from build123d import *

# Parameters (mm, degrees)
SKETCH1_R           = 25
BOSS_EXTRUDE1_DEPTH = 15
CUT_EXTRUDE1_DEPTH  = 150
SKETCH3_R           = 1.5
CUT_EXTRUDE2_DEPTH  = 44.660622991
CUT_EXTRUDE3_START  = -7.5
SKETCH4_R           = 2.5
CUT_EXTRUDE3_DEPTH  = 10
CIRPATTERN1_COUNT   = 3
SKETCH5_R           = 2.5
CUT_EXTRUDE4_DEPTH  = 39.405728909


with BuildPart() as part:
    # Sketch1 → Boss-Extrude1 (new body)
    with BuildSketch(Plane(origin=(0, 0, 0), x_dir=(1, 0, 0), z_dir=(0, 1, 0))):
        with Locations(Location((0, 0, 0), (0, 0, 270))):
            Circle(SKETCH1_R)
    extrude(amount=BOSS_EXTRUDE1_DEPTH)

    # Sketch2 → Cut-Extrude1 (cut)
    with BuildSketch(Plane(origin=(0, 15, 0), x_dir=(1, 0, 0), z_dir=(0, 1, 0))):
        with BuildLine():
            Line((7.5, -10), (-7.5, -10))
            Line((-7.5, -10), (-7.5, -23.848480035))
            ThreePointArc((-7.5, -23.848480035), (0, -25), (7.5, -23.848480035))
            Line((7.5, -23.848480035), (7.5, -10))
        make_face()
    cut_extrude1 = extrude(amount=-CUT_EXTRUDE1_DEPTH, mode=Mode.SUBTRACT)

    # Sketch3 → Cut-Extrude2 (cut, symmetric)
    with BuildSketch(Plane.ZY.offset(-7.5)):
        with Locations((16.924240018, 7.5)):
            Circle(SKETCH3_R)
    cut_extrude2 = extrude(amount=CUT_EXTRUDE2_DEPTH, both=True, mode=Mode.SUBTRACT)

    # Sketch4 → Cut-Extrude3 (cut)
    with BuildSketch(Plane.ZY.offset(-7.5).offset(CUT_EXTRUDE3_START)):
        with Locations((16.924240018, 7.5)):
            Circle(SKETCH4_R)
    cut_extrude3 = extrude(amount=-CUT_EXTRUDE3_DEPTH, mode=Mode.SUBTRACT)

    # CirPattern1: Cut-Extrude1, Cut-Extrude2, Cut-Extrude3 ×3 about axis
    cirpattern1_axis = Axis((0, 0, 0), (0, 1, 0))
    add([cut_extrude1.rotate(cirpattern1_axis, i * 360 / CIRPATTERN1_COUNT) for i in range(1, CIRPATTERN1_COUNT)], mode=Mode.SUBTRACT)
    add([cut_extrude2.rotate(cirpattern1_axis, i * 360 / CIRPATTERN1_COUNT) for i in range(1, CIRPATTERN1_COUNT)], mode=Mode.SUBTRACT)
    add([cut_extrude3.rotate(cirpattern1_axis, i * 360 / CIRPATTERN1_COUNT) for i in range(1, CIRPATTERN1_COUNT)], mode=Mode.SUBTRACT)

    # Sketch5 → Cut-Extrude4 (cut, through all)
    with BuildSketch(Plane(origin=(0, 15, 0), x_dir=(1, 0, 0), z_dir=(0, 1, 0))):
        with Locations(Location((0, 0, 0), (0, 0, 270))):
            Circle(SKETCH5_R)
    extrude(amount=-CUT_EXTRUDE4_DEPTH, mode=Mode.SUBTRACT)


solid = part.part
Could you check a few things on this model? Use its own coordinates, in mm. A direction names the side the tool comes from. Round coordinates to 2 decimals unless told otherwise and drop trailing zeros. Write each loop counter-clockwise with the first axis right and the second up, starting at its lowest first coordinate (ties: lowest second). Pieces come first, ordered by that corner, then holes. Notation, with made-up numbers: (-15, -40) - (-11, -40) arc R23 ccw to (-11, -7) - close; hole circle Ø6 at (-22.75, 33.5). An arc over 180 degrees is marked (long way). Put each result on its own line as item: value. Start each with the question number.
(1) I want a section at A-A, the plane x = 0. Please give me the cut outline in (y, z), plus the area to 3 significant figures.
(2) I need wall thicknesses on probe 1 along X at (y, z) = (10, 0); probe 2 along X at (y, z) = (11.5, 16); probe 3 along Z at (x, y) = (-20, 6.5). Which ranges of each line are inside material? Lowest first, please.
(3) Thinking about a two-plate mould opening in Y: for faces 5 (the flat face through (0, 0, 5)), 6 (the cylindrical face through (3.959, 7.61, -21.996)), 7 (the flat face through (-7.5, 8, 15)), which applies, released by +Y, released by -Y, zero draft, split by the parting line, or undercut?
(4) Will these pins go through, and if not, where does the flat tip stop? pin 1 (4 mm diameter, centred on y = 7, z = 1, fed in from +X); pin 2 (2 mm diameter, centred on y = 7.5, z = 13.5, fed in from +X); pin 3 (1.8 mm diameter, centred on y = 7.5, z = 16.92, fed in from -X); pin 4 (2 mm diameter, centred on x = -6.5, y = 6, fed in from -Z).
(5) I want a section at C-C, the plane z = 16.5. Please give me the cut outline in (x, y).
(6) I want a section at D-D, the plane y = 7.5. Give the number of separate pieces and of enclosed holes in the cut face, plus the area to 3 significant figures.
(7) I want a section at B-B, the plane y = 13.5. Please give me the cut outline in (x, z), plus the area to 3 significant figures.
(8) For faces 1 (the flat face through (8.57, 6.98, -22.27)), 2 (the cylindrical face through (17.07, 7.61, 14.427)), 3 (the flat face through (8.61, 7.6, -5.09)), 4 (the flat face through (10.991, 9.272, -15.006)), which set-ups out of +Z, -Z, +X, -X, +Y, -Y let a thin tool reach every point of the face, with its end or its side?
Here are the results:
1. outline: (0, -25) - (15, -25) - (15, -2.5) - (0, -2.5) - close; (0, 2.5) - (15, 2.5) - (15, 10) - (0, 10) - close
1. area: 450 mm^2
2. probe 1: x = -25 to -15, -11.55 to -2.5, 2.5 to 11.55, 15 to 25
2. probe 2: x = -19.21 to -7.5, 7.5 to 19.21
2. probe 3: z = -2.89 to -1.44, 3.03 to 15
3. face 5: released by -Y
3. face 6: undercut
3. face 7: zero draft
4. pin 1: stops at x = 25
4. pin 2: stops at x = 21.65
4. pin 3: passes through
4. pin 4: stops at z = -24.39
5. outline: (-18.78, 0) - (-7.5, 0) - (-7.5, 6.06) - (-18.78, 6.06) - close; (-18.78, 8.94) - (-7.5, 8.94) - (-7.5, 15) - (-18.78, 15) - close; (7.5, 0) - (18.78, 0) - (18.78, 5.04) - (15, 5.04) - (15, 6.06) - (7.5, 6.06) - close; (7.5, 8.94) - (15, 8.94) - (15, 9.96) - (18.78, 9.96) - (18.78, 15) - (7.5, 15) - close
6. separate pieces: 7
6. enclosed holes: 1
6. area: 1,070 mm^2
7. outline: (-24.4, -5.43) - (-12.41, 1.5) - (-4.91, -11.5) - (-16.9, -18.42) arc R25 ccw to (16.9, -18.42) - (4.91, -11.5) - (12.41, 1.5) - (24.4, -5.43) arc R25 ccw to (7.5, 23.85) - (7.5, 10) - (-7.5, 10) - (-7.5, 23.85) arc R25 ccw to start; hole circle Ø5 at (0, 0)
7. area: 1,290 mm^2
8. face 1: none
8. face 2: +X
8. face 3: +Y, -Y
8. face 4: +X, +Y, -Y
